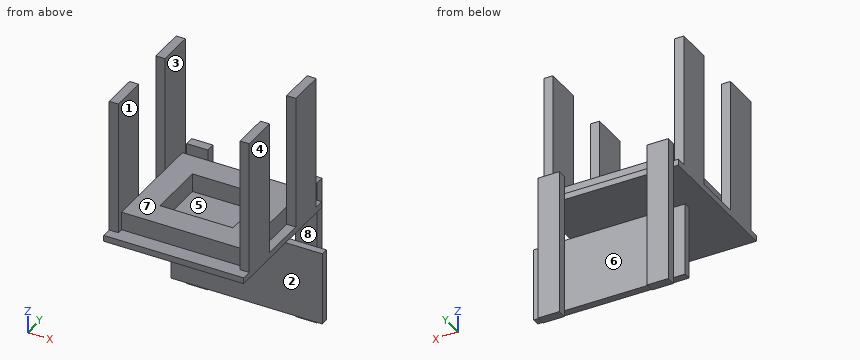
```python
from build123d import *

# Parameters (mm, degrees)
F0_W           = 292.1
F0_H           = 292.1
F1_DEPTH       = 12.7
F3_W           = 19.05
F3_H           = 76.2
F4_DEPTH       = 279.4
F6_W           = 53.0352
F6_H           = 38.1
F7_DEPTH       = 254
F9_W           = 50.8
F9_H           = 38.1
F10_DEPTH      = 121.8899004574
F11_W          = 44.45
F11_H          = 19.05
F12_DEPTH      = 254
F12_DEPTH_BACK = 49.89103
F13_W          = 19.8010608381
F13_H          = 152.4
F13_W_2        = 44.45
F13_W_3        = 251.7297603481
F14_DEPTH      = 15.24


with BuildPart() as f1:
    # F0 (on Top) → F1 (new body)
    with BuildSketch(Plane.XY):
        with Locations((-9.5041804016, 32.6594091807)):
            Rectangle(F0_W, F0_H)
    extrude(amount=-F1_DEPTH)

    # F3 (on face) → F4 (join)
    with BuildSketch(Plane.XY):
        with Locations((127.0208195984, -54.4418936728)):
            Rectangle(F3_W, F3_H)
        with Locations((127.0208195984, 119.7607120342)):
            Rectangle(F3_W, F3_H)
        with Locations((-146.0291804016, -54.4418936728)):
            Rectangle(F3_W, F3_H)
        with Locations((-146.0291804016, 119.7607120342)):
            Rectangle(F3_W, F3_H)
    extrude(amount=F4_DEPTH)

    # F6 (on face) → F7 (join, through all)
    with BuildSketch(Plane(origin=(117.4958195984, 0, 0), x_dir=(0, -1, 0), z_dir=(-1, 0, 0))):
        with Locations((54.4418936728, 19.05)):
            Rectangle(F6_W, F6_H)
        with Locations((-120.4832067846, 19.05)):
            Rectangle(F6_W, F6_H)
    extrude(amount=F7_DEPTH)

    # F9 (on face) → F10 (join, through all)
    with BuildSketch(Plane(origin=(0, -27.9242936728, 0), x_dir=(-1, 0, 0), z_dir=(0, 1, 0))):
        with Locations((-92.0958195984, 19.05)):
            Rectangle(F9_W, F9_H)
        with Locations((111.1041804016, 19.05)):
            Rectangle(F9_W, F9_H)
    extrude(amount=F10_DEPTH)

    # F11 (on face) → F12 (join, two sides)
    with BuildSketch(Plane(origin=(0, 0, -12.7), x_dir=(1, 0, 0), z_dir=(0, 0, -1))) as f12_sk:
        with Locations((104.1608195984, -188.2344091807)):
            Rectangle(F11_W, F11_H)
        with Locations((-123.1691804016, -188.2344091807)):
            Rectangle(F11_W, F11_H)
    extrude(amount=F12_DEPTH)
    extrude(f12_sk.sketch, amount=-F12_DEPTH_BACK)

    # F13 (on face) → F14 (join)
    with BuildSketch(Plane.XZ.offset(-178.7094091807)):
        with Locations((136.2863500175, -177.8)):
            Rectangle(F13_W, F13_H)
        with Locations((104.1608195984, -177.8)):
            Rectangle(F13_W_2, F13_H)
        with Locations((-43.9290605756, -177.8)):
            Rectangle(F13_W_3, F13_H)
    extrude(amount=F14_DEPTH)


solid = f1.part
```
Work out the finished part from the listing and answer in its coordinate system (mm). Face numbers are marked on the shaded views. A direction names the side the tool comes from. Round coordinates to 2 decimals unless told otherwise and drop trailing zeros. Loops run counter-clockwise (first coordinate to the right, second up) from the corner with the lowest first, then second, coordinate; pieces in that order, holes last. Notation, with made-up numbers: M 2.5,-33.75 L 11.5,-33.75 A23 ccw 11.5,-14.75 Z; hole C -18.75,34 d8. An arc over 180 degrees is marked long. One line per question, with ' | ' between items.
Q1. Find section B-B, the plane x = -18. Give the vertices of the cut face in (y, z).
Conclusion:
outline: M -113.39,-12.7 L 178.71,-12.7 L 178.71,0 L 147,0 L 147,38.1 L 93.97,38.1 L 93.97,0 L -27.92,0 L -27.92,38.1 L -80.96,38.1 L -80.96,0 L -113.39,0 Z; M 163.47,-254 L 178.71,-254 L 178.71,-101.6 L 163.47,-101.6 Z
Q2. Consider line 1 along X through (y, z) = (-54, 50); line 2 along Y through (x, z) = (49, -166); line 3 along Z through (x, y) = (-146, -47.5). Determine where each line is inside the solid, lowest interval first. Write a range as from..to.
Conclusion:
line 1: x = -155.55..-136.5, 117.5..136.55 | line 2: y = 163.47..178.71 | line 3: z = -12.7..279.4
Q3. Find section D-D, the plane y = 19.5. Give the vertices of the cut face in (x, z), then the cut area to 3 significant figures.
Conclusion:
outline: M -155.55,-12.7 L 136.55,-12.7 L 136.55,0 L 117.5,0 L 117.5,38.1 L 66.7,38.1 L 66.7,0 L -85.7,0 L -85.7,38.1 L -136.5,38.1 L -136.5,0 L -155.55,0 Z | area: 7,580 mm2
Q4. Find section C-C, the plane z = -27.5. Give the vertices of the cut face in (x, y).
Conclusion:
outline: M -145.39,178.71 L -100.94,178.71 L -100.94,197.76 L -145.39,197.76 Z; M 81.94,178.71 L 126.39,178.71 L 126.39,197.76 L 81.94,197.76 Z
Q5. Each of these flat-tipped pins is pushed along its axis until it touches: pin 1 Ø1 at (y, z) = (-17.5, 32) entering from +X; pin 2 Ø12 at (x, y) = (-26.5, 174) entering from +Z; pin 3 Ø9.5 at (x, z) = (-144.5, 82.5) entering from +Y. Where does it stop, or does it pass through?
Conclusion:
pin 1: stops at x = 136.55 | pin 2: stops at z = 0 | pin 3: stops at y = 157.86
Q6. The mould has two halves that part along X. Classify the marked faces 1, 2, 3 and 4: +X half, -X half, draft (parallel to the pull), parting line (faces both ways), or undercut.
Conclusion:
face 1: undercut | face 2: draft | face 3: undercut | face 4: +X half
Q7. Find section A-A, the plane z = 57.5. Give the vertices of the cut face in (x, y).
Conclusion:
outline: M -155.55,-92.54 L -136.5,-92.54 L -136.5,-16.34 L -155.55,-16.34 Z; M -155.55,81.66 L -136.5,81.66 L -136.5,157.86 L -155.55,157.86 Z; M 117.5,-92.54 L 136.55,-92.54 L 136.55,-16.34 L 117.5,-16.34 Z; M 117.5,81.66 L 136.55,81.66 L 136.55,157.86 L 117.5,157.86 Z
Q8. A tool of negligible diameter and unlimited length cuts with its end or side. For the marked faces 5, 6, 7 and 8, from which of +Z, -Z, +X, -X, +Y, -Y can it reach the whole face along a straight path? Write none if from no direction.
Conclusion:
face 5: +Z | face 6: +Z, -Z, +Y | face 7: +Z, +Y, -Y | face 8: +X, -X, -Y
